from build123d import *

# Parameters (mm, degrees)
F0_W         = 38
F0_H         = 22
F0_R         = 1.5
F0_W_2       = 23
F0_H_2       = 14.5
F1_DEPTH     = 2.75
F2_R         = 1
F3_T3_ANGLE  = 90
F3_T6_ANGLE  = 90
F3_T9_ANGLE  = 90
F3_T12_ANGLE = 90
F3_T15_DEPTH = 15.2524142536
F3_T18_DEPTH = 15.2524142536
F3_T21_DEPTH = 15.2524142536
F3_T24_DEPTH = 15.2524142536


# Not quite as in the source:
# - a fillet or chamfer that OpenCascade refuses, or shapes differently, is made with other operations: its cross-section is extruded or revolved along the edge and cut away or added


with BuildPart() as f1:
    # F0 (on Top) → F1 (new body)
    with BuildSketch(Plane.XY):
        with Locations((0.1353118792, -1.2320824713)):
            Rectangle(F0_W, F0_H)
        with Locations((-13.6146881208, -1.2320824713)):
            Circle(F0_R, mode=Mode.SUBTRACT)
        with Locations((0.1353118792, -1.2320824713)):
            Rectangle(F0_W_2, F0_H_2, mode=Mode.SUBTRACT)
        with Locations((13.8853118792, -1.2320824713)):
            Circle(F0_R, mode=Mode.SUBTRACT)
    extrude(amount=F1_DEPTH)

    # F2
    f2_edges = [f1.edges().sort_by_distance(p)[0] for p in [
        (19.135312, -1.232082, 0),
        (0.135312, 9.767918, 0),
        (-18.864688, -1.232082, 0),
        (0.135312, -12.232082, 0),
    ]]
    fillet(f2_edges, radius=F2_R)

    # F3: fillet of radius 5 on 4 edges, made by hand


with BuildPart() as f3_tool1:
    # F3_s2 → F3_t3 (revolve)
    with BuildSketch(Plane.XZ.offset(-4.7669518433)):
        with BuildLine():
            ThreePointArc((-17.8650881208, 0), (-18.572194902, 0.2928932188), (-18.8650881208, 1))
            Line((-18.8650881208, 1), (-18.8650881208, 0))
            Line((-18.8650881208, 0), (-17.8650881208, 0))
        make_face()
    revolve(axis=Axis((-13.8637224354, 4.7669518433, 0), (0, 0, -1)), revolution_arc=F3_T3_ANGLE)


with BuildPart() as f3_tool4:
    # F3_s5 → F3_t6 (revolve)
    with BuildSketch(Plane.YZ.offset(-13.8637224354)):
        with BuildLine():
            ThreePointArc((-11.2324824713, 0), (-11.9395892524, 0.2928932188), (-12.2324824713, 1))
            Line((-12.2324824713, 1), (-12.2324824713, 0))
            Line((-12.2324824713, 0), (-11.2324824713, 0))
        make_face()
    revolve(axis=Axis((-13.8637224354, -7.2311167858, 0), (0, 0, -1)), revolution_arc=F3_T6_ANGLE)


with BuildPart() as f3_tool7:
    # F3_s8 → F3_t9 (revolve)
    with BuildSketch(Plane.XZ.offset(7.2311167858)):
        with BuildLine():
            ThreePointArc((18.1357118792, 0), (18.8428186604, 0.2928932188), (19.1357118792, 1))
            Line((19.1357118792, 1), (19.1357118792, 0))
            Line((19.1357118792, 0), (18.1357118792, 0))
        make_face()
    revolve(axis=Axis((14.1343461938, -7.2311167858, 0), (0, 0, -1)), revolution_arc=F3_T9_ANGLE)


with BuildPart() as f3_tool10:
    # F3_s11 → F3_t12 (revolve)
    with BuildSketch(Plane.YZ.offset(14.1343461938)):
        with BuildLine():
            ThreePointArc((8.7683175287, 0), (9.4754243099, 0.2928932188), (9.7683175287, 1))
            Line((9.7683175287, 1), (9.7683175287, 0))
            Line((9.7683175287, 0), (8.7683175287, 0))
        make_face()
    revolve(axis=Axis((14.1343461938, 4.7669518433, 0), (0, 0, -1)), revolution_arc=F3_T12_ANGLE)


with BuildPart() as f3_tool13:
    # F3_s14 → F3_t15 (new body)
    with BuildSketch(Plane.XY):
        with BuildLine():
            ThreePointArc((14.1343461938, 9.7683175287), (17.6708457852, 8.3034514347), (19.1357118792, 4.7669518433))
            Line((19.1357118792, 4.7669518433), (19.6358484478, 4.7669518433))
            ThreePointArc((19.6358484478, 4.7669518433), (19.6354484478, 7.267434686), (19.6354484478, 9.7679175287))
            Line((19.6354484478, 9.7679175287), (19.1353118792, 10.2680540973))
            ThreePointArc((19.1353118792, 10.2680540973), (16.6348290365, 10.2680540973), (14.1343461938, 10.2684540973))
            Line((14.1343461938, 10.2684540973), (14.1343461938, 9.7683175287))
        make_face()
    extrude(amount=F3_T15_DEPTH)


with BuildPart() as f3_tool16:
    # F3_s17 → F3_t18 (new body)
    with BuildSketch(Plane.XY):
        with BuildLine():
            ThreePointArc((19.1357118792, -7.2311167858), (17.6708457852, -10.7676163772), (14.1343461938, -12.2324824713))
            Line((14.1343461938, -12.2324824713), (14.1343461938, -12.7326190398))
            ThreePointArc((14.1343461938, -12.7326190398), (16.6348290365, -12.7322190398), (19.1353118792, -12.7322190398))
            Line((19.1353118792, -12.7322190398), (19.6354484478, -12.2320824713))
            ThreePointArc((19.6354484478, -12.2320824713), (19.6354484478, -9.7315996285), (19.6358484478, -7.2311167858))
            Line((19.6358484478, -7.2311167858), (19.1357118792, -7.2311167858))
        make_face()
    extrude(amount=F3_T18_DEPTH)


with BuildPart() as f3_tool19:
    # F3_s20 → F3_t21 (new body)
    with BuildSketch(Plane.XY):
        with BuildLine():
            ThreePointArc((-18.8650881208, -7.2311167858), (-17.4002220267, -10.7676163772), (-13.8637224354, -12.2324824713))
            Line((-13.8637224354, -12.2324824713), (-13.8637224354, -12.7326190398))
            ThreePointArc((-13.8637224354, -12.7326190398), (-16.3642052781, -12.7322190398), (-18.8646881208, -12.7322190398))
            Line((-18.8646881208, -12.7322190398), (-19.3648246893, -12.2320824713))
            ThreePointArc((-19.3648246893, -12.2320824713), (-19.3648246893, -9.7315996285), (-19.3652246893, -7.2311167858))
            Line((-19.3652246893, -7.2311167858), (-18.8650881208, -7.2311167858))
        make_face()
    extrude(amount=F3_T21_DEPTH)


with BuildPart() as f3_tool22:
    # F3_s23 → F3_t24 (new body)
    with BuildSketch(Plane.XY):
        with BuildLine():
            ThreePointArc((-13.8637224354, 9.7683175287), (-17.4002220267, 8.3034514347), (-18.8650881208, 4.7669518433))
            Line((-18.8650881208, 4.7669518433), (-19.3652246893, 4.7669518433))
            ThreePointArc((-19.3652246893, 4.7669518433), (-19.3648246893, 7.267434686), (-19.3648246893, 9.7679175287))
            Line((-19.3648246893, 9.7679175287), (-18.8646881208, 10.2680540973))
            ThreePointArc((-18.8646881208, 10.2680540973), (-16.3642052781, 10.2680540973), (-13.8637224354, 10.2684540973))
            Line((-13.8637224354, 10.2684540973), (-13.8637224354, 9.7683175287))
        make_face()
    extrude(amount=F3_T24_DEPTH)


with BuildPart() as f1_1:
    add(f1.part)

    # F3_t25: cut F3_tool1, F3_tool4, F3_tool7, F3_tool10, F3_tool13, F3_tool16, F3_tool19, F3_tool22
    add([f3_tool1.part, f3_tool4.part, f3_tool7.part, f3_tool10.part, f3_tool13.part, f3_tool16.part, f3_tool19.part, f3_tool22.part], mode=Mode.SUBTRACT)


solid = f1_1.part
Design review of the part built by this model. Coordinates are the model's own, in mm. A direction names the side the tool comes from. Round coordinates to 2 decimals unless told otherwise and drop trailing zeros. Write each loop counter-clockwise with the first axis right and the second up, starting at its lowest first coordinate (ties: lowest second). Pieces come first, ordered by that corner, then holes.
Item 1: For pin 1 Ø12 at (x, y) = (-1.5, -3.5) entering from -Z, flat-tipped, find the tip position at first contact; note if it passes through.
Item 2: Draft analysis for pull direction X (two halves, no side actions). For faces 3 (the cylindrical face through (17.632, 8.342, 1.863)), 4 (the flat face through (0, 9.768, 2)), 5 (the flat face through (-11.365, -1, 1)), 6 (the cylindrical face through (15.27, -1.81, 1.36)), state which applies: released by +X, released by -X, zero draft, split by the parting line, or undercut.
Item 3: Consider section C-C on y = -2.25. Give the boundary of the cut face in (x, z).
Item 4: Consider section B-B on x = 10.5. Give the boundary of the cut face in (y, z), and give its area (3 significant figures).
Item 5: For faces 1 (the flat face through (0, -8.482, 1)), 2 (the flat face through (19.135, -1, 2)), list the 3-axis set-ups (+Z, -Z, +X, -X, +Y, -Y) from which the entire face can be reached by the end or side of a thin tool; tool diameter is ignored.
Item 6: Consider section A-A on y = -5.5. Give the boundary of the cut face in (x, z).
Item 7: Wall thickness on L1, parallel to X at y = -6.5, z = 2.15; L2, parallel to Y at x = -10, z = 1.3; L3, parallel to X at y = -2, z = 0.5: over which ranges is each line inside the solid? List them lowest first.
Item 8: Consider section D-D on z = 1.9. Give the boundary of the cut face in (x, y), and give its area (3 significant figures).
Check values:
1. pin 1: stops at z = 0
2. face 3: released by +X
2. face 4: zero draft
2. face 5: undercut
2. face 6: undercut
3. outline: (-18.86, 1) arc R1 ccw to (-17.86, 0) - (-14.72, 0) - (-14.72, 2.75) - (-18.86, 2.75) - close; (-12.51, 0) - (-11.36, 0) - (-11.36, 2.75) - (-12.51, 2.75) - close; (11.64, 0) - (12.78, 0) - (12.78, 2.75) - (11.64, 2.75) - close; (14.99, 0) - (18.14, 0) arc R1 ccw to (19.14, 1) - (19.14, 2.75) - (14.99, 2.75) - close
4. outline: (-12.23, 1) arc R1 ccw to (-11.23, 0) - (-8.48, 0) - (-8.48, 2.75) - (-12.23, 2.75) - close; (6.02, 0) - (8.77, 0) arc R1 ccw to (9.77, 1) - (9.77, 2.75) - (6.02, 2.75) - close
4. area: 20.2 mm2
5. face 1: +Z, -Z
5. face 2: +Z, -Z, +X, +Y, -Y
6. outline: (-18.86, 1) arc R1 ccw to (-17.86, 0) - (-11.36, 0) - (-11.36, 2.75) - (-18.86, 2.75) - close; (11.64, 0) - (18.14, 0) arc R1 ccw to (19.14, 1) - (19.14, 2.75) - (11.64, 2.75) - close
7. L1: x = -18.86 to -11.36, 11.64 to 19.14
7. L2: y = -12.23 to -8.48, 6.02 to 9.77
7. L3: x = -18.73 to -14.9, -12.33 to -11.36, 11.64 to 12.6, 15.17 to 19
8. outline: (-18.86, -7.29) arc R5 ccw to (-13.93, -12.23) - (14.2, -12.23) arc R5 ccw to (19.14, -7.29) - (19.14, 4.83) arc R5 ccw to (14.2, 9.77) - (-13.93, 9.77) arc R5 ccw to (-18.86, 4.83) - close; hole circle Ø3 at (-13.61, -1.23); hole (-11.36, -8.48) - (11.64, -8.48) - (11.64, 6.02) - (-11.36, 6.02) - close; hole circle Ø3 at (13.89, -1.23)
8. area: 467 mm2
